from build123d import *

# Parameters (mm, degrees)
SKETCH1_R           = 40.5
BOSS_EXTRUDE1_DEPTH = 2
SKETCH2_R           = 1.5
CUT_EXTRUDE1_DEPTH  = 2
SKETCH3_R           = 7.5
CUT_EXTRUDE2_DEPTH  = 2


with BuildPart() as part:
    # Sketch1 → Boss-Extrude1 (new body)
    with BuildSketch(Plane(origin=(0, 0, 0), x_dir=(1, 0, 0), z_dir=(0, 1, 0))):
        with Locations(Location((0, 0, 0), (0, 0, 270))):
            Circle(SKETCH1_R)
    extrude(amount=BOSS_EXTRUDE1_DEPTH)

    # Sketch2 → Cut-Extrude1 (cut)
    with BuildSketch(Plane(origin=(0, 2, 0), x_dir=(1, 0, 0), z_dir=(0, 1, 0))):
        with Locations(Location((0, 38, 0), (0, 0, 270))):
            Circle(SKETCH2_R)
        with Locations(Location((38, 0, 0), (0, 0, 270))):
            Circle(SKETCH2_R)
        with Locations(Location((0, -38, 0), (0, 0, 270))):
            Circle(SKETCH2_R)
    extrude(amount=-CUT_EXTRUDE1_DEPTH, mode=Mode.SUBTRACT)

    # Sketch3 → Cut-Extrude2 (cut)
    with BuildSketch(Plane(origin=(0, 2, 0), x_dir=(1, 0, 0), z_dir=(0, 1, 0))):
        with Locations(Location((0, 0, 0), (0, 0, 270))):
            Circle(SKETCH3_R)
    extrude(amount=-CUT_EXTRUDE2_DEPTH, mode=Mode.SUBTRACT)


solid = part.part
Read the model definition and answer for the solid it produces. Units are mm, in the model's axes. Coordinates: 2 decimals unless noted, no trailing zeros. Loops run counter-clockwise (first coordinate to the right, second up) from the corner with the lowest first, then second, coordinate; pieces in that order, holes last. Notation, with made-up numbers: (-22.5, 26.5) - (23.5, 26.5) arc R28 cw to (23.5, 46.5) - close; hole circle Ø9 at (63, -17.75). An arc over 180 degrees is marked (long way). Answer in a Markdown table with one row per item.
Q1. The mould has two halves that part along Z. Classify faces 1 (the cylindrical face through (34.15, 0.99, 21.77)), 2 (the cylindrical face through (0.33, 1.014, -7.493)), 3 (the flat face through (-8, 2, -1)): pulls with the +Z half, pulls with the -Z half, needs draft (parallel to the pull), parting line crosses it, or undercut.
Here are the results:
| item | result |
|---|---|
| face 1 | parting line crosses it |
| face 2 | undercut |
| face 3 | needs draft |
Q2. Find section C-C on y = 0.3. Write down the section's boundary in (x, z).
Here are the results:
| item | result |
|---|---|
| outline | circle Ø81 at (0, 0); hole circle Ø15 at (0, 0); hole circle Ø3 at (0, -38); hole circle Ø3 at (0, 38); hole circle Ø3 at (38, 0) |
Q3. Straight lines are drawn through the part: line 1 along X through (y, z) = (1.2, 0); line 2 along X through (y, z) = (0.8, -9). For each, find the intervals that lie inside material, in ascending order. Write a range as [from, to].
Here are the results:
| item | result |
|---|---|
| line 1 | x = [-40.5, -7.5], [7.5, 36.5], [39.5, 40.5] |
| line 2 | x = [-39.49, 39.49] |
Q4. Find section D-D on z = 38. Write down the section's boundary in (x, y), plus the area to 3 significant figures.
Here are the results:
| item | result |
|---|---|
| outline | (-14.01, 0) - (-1.5, 0) - (-1.5, 2) - (-14.01, 2) - close; (1.5, 0) - (14.01, 0) - (14.01, 2) - (1.5, 2) - close |
| area | 50.0 mm^2 |
Q5. Find section B-B on z = 0. Write down the section's boundary in (x, y), plus the area to 3 significant figures.
Here are the results:
| item | result |
|---|---|
| outline | (-40.5, 0) - (-7.5, 0) - (-7.5, 2) - (-40.5, 2) - close; (7.5, 0) - (36.5, 0) - (36.5, 2) - (7.5, 2) - close; (39.5, 0) - (40.5, 0) - (40.5, 2) - (39.5, 2) - close |
| area | 126 mm^2 |
Q6. Find section A-A on x = 0. Write down the section's boundary in (y, z), plus the area to 3 significant figures.
Here are the results:
| item | result |
|---|---|
| outline | (0, -40.5) - (2, -40.5) - (2, -39.5) - (0, -39.5) - close; (0, -36.5) - (2, -36.5) - (2, -7.5) - (0, -7.5) - close; (0, 7.5) - (2, 7.5) - (2, 36.5) - (0, 36.5) - close; (0, 39.5) - (2, 39.5) - (2, 40.5) - (0, 40.5) - close |
| area | 120 mm^2 |
